Input: part model. Units: mm. Frame: model coordinates. Face numbers are marked on the shaded views. A direction names the side the tool comes from. Coordinates: 2 decimals unless noted, no trailing zeros. Write each loop counter-clockwise with the first axis right and the second up, starting at its lowest first coordinate (ties: lowest second). Pieces come first, ordered by that corner, then holes.
1) Pin query (flat end, axial travel): pin 1 Ø0.9 at (x, y) = (-39.5, 23) entering from +Z; pin 2 Ø2 at (y, z) = (-8.5, 6) entering from +X; pin 3 Ø0.6 at (y, z) = (42, 1) entering from +X. Return the tip coordinate at first contact, or that it passes through.
2) Section query C-C (z = 10.5). Output: boundary loops of the cut face in (x, y), then the cut area to 3 significant figures.
3) Section query D-D (y = 33.5). Output: boundary loops of the cut face in (x, z), then the cut area to 3 significant figures.
4) Set-up query: the marked faces 1 and 2. Return all of +Z, -Z, +X, -X, +Y, -Y with unobstructed straight access to the full face (end or side cutting, diameter ignored); none if empty.
5) Section query A-A (x = 0). Output: boundary loops of the cut face in (y, z), then the cut area to 3 significant figures.
6) Line query: L1, parallel to Z at x = 40, y = 0; L2, parallel to Y at x = -26, z = 1.75; L3, parallel to X at y = 5.5, z = 6.75. Output: solid intervals per line, ascending.
Autodesk Fusion 360 part; units mm, degrees
sketch "Sketch1" plane through (0, 0, 0) normal (0, 0, 1) x (1, 0, 0)
  circle A0 centre (0, 0) radius 38.1
  circle A1 centre (0, 0) radius 46 construction
  circle A2 centre (0, 46) radius 4
  line L0 (-3.9962, 45.8261) -> (-3.9962, 37.8898)
  line L1 (3.9962, 45.8261) -> (3.9962, 37.8898)
  circle A3 centre (0, 46) radius 1.5
  line L2 (-19.4522, 41.6847) -> (-15.4841, 34.8117)
  line L3 (-26.3739, 37.6884) -> (-22.4057, 30.8155)
  circle A4 centre (-23, 39.8372) radius 4
  circle A5 centre (-23, 39.8372) radius 1.5
  line L4 (-37.6884, 26.3739) -> (-30.8155, 22.4057)
  line L5 (-41.6847, 19.4522) -> (-34.8117, 15.4841)
  circle A6 centre (-39.8372, 23) radius 4
  circle A7 centre (-39.8372, 23) radius 1.5
  line L6 (-45.8261, 3.9962) -> (-37.8898, 3.9962)
  line L7 (-45.8261, -3.9962) -> (-37.8898, -3.9962)
  circle A8 centre (-46, 0) radius 4
  circle A9 centre (-46, 0) radius 1.5
  line L8 (-41.6847, -19.4522) -> (-34.8117, -15.4841)
  line L9 (-37.6884, -26.3739) -> (-30.8155, -22.4057)
  circle A10 centre (-39.8372, -23) radius 4
  circle A11 centre (-39.8372, -23) radius 1.5
  line L10 (-26.3739, -37.6884) -> (-22.4057, -30.8155)
  line L11 (-19.4522, -41.6847) -> (-15.4841, -34.8117)
  circle A12 centre (-23, -39.8372) radius 4
  circle A13 centre (-23, -39.8372) radius 1.5
  line L12 (-3.9962, -45.8261) -> (-3.9962, -37.8898)
  line L13 (3.9962, -45.8261) -> (3.9962, -37.8898)
  circle A14 centre (0, -46) radius 4
  circle A15 centre (0, -46) radius 1.5
  line L14 (19.4522, -41.6847) -> (15.4841, -34.8117)
  line L15 (26.3739, -37.6884) -> (22.4057, -30.8155)
  circle A16 centre (23, -39.8372) radius 4
  circle A17 centre (23, -39.8372) radius 1.5
  line L16 (37.6884, -26.3739) -> (30.8155, -22.4057)
  line L17 (41.6847, -19.4522) -> (34.8117, -15.4841)
  circle A18 centre (39.8372, -23) radius 4
  circle A19 centre (39.8372, -23) radius 1.5
  line L18 (45.8261, -3.9962) -> (37.8898, -3.9962)
  line L19 (45.8261, 3.9962) -> (37.8898, 3.9962)
  circle A20 centre (46, 0) radius 4
  circle A21 centre (46, 0) radius 1.5
  line L20 (41.6847, 19.4522) -> (34.8117, 15.4841)
  line L21 (37.6884, 26.3739) -> (30.8155, 22.4057)
  circle A22 centre (39.8372, 23) radius 4
  circle A23 centre (39.8372, 23) radius 1.5
  line L22 (26.3739, 37.6884) -> (22.4057, 30.8155)
  line L23 (19.4522, 41.6847) -> (15.4841, 34.8117)
  circle A24 centre (23, 39.8372) radius 4
  circle A25 centre (23, 39.8372) radius 1.5
  dimension "d374" = 76.2
  dimension "d375" = 92
  dimension "d376" = 8
  dimension "d377" = 3
  dimension "d379" = 360
extrude "Extrude1" add sketch "Sketch1" along normal blind 2 contours A0 | A0 L18 L19 A20 | A0 L20 L21 A22 | A20 | A0 L16 L17 A18 | A22 | A18 | A0 L22 L23 A24 | A0 L14 L15 A16 | A24 | A16 | A0 A2 L0 L1 | A0 L12 L13 A14 | A2 | A14 | A0 L2 L3 A4 | A0 L10 L11 A12 | A4 | A12 | A0 L4 L5 A6 | A0 L8 L9 A10 | A6 | A10 | A0 L6 L7 A8 | A8 | A3 | A5 | A7 | A9 | A11 | A13 | A15 | A17 | A19 | A21 | A23 | A25
extrude "Extrude2" add sketch "Sketch1" along normal blind 10 from surface at 2 contours A0
extrude "Extrude3" add sketch "Sketch1" along normal blind 3 from surface at 2 contours A3 | A5 | A7 | A9 | A11 | A13 | A15 | A17 | A19 | A21 | A23 | A25
equation "d374 = mmt_id"
equation "mmt_id = 76.2 mm"
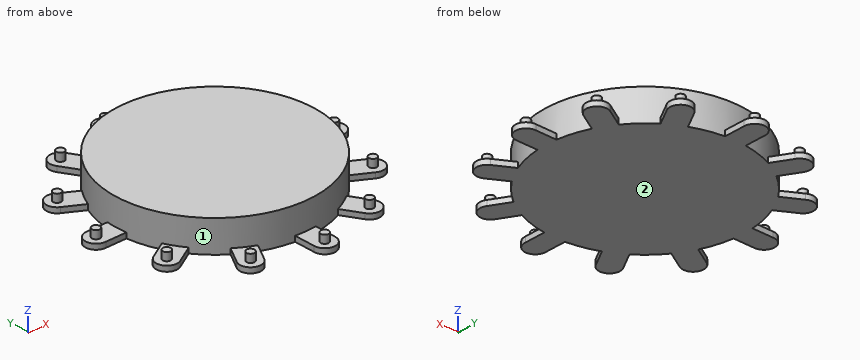
Answer:
1. pin 1: stops at z = 5
1. pin 2: stops at x = 37.35
1. pin 3: stops at x = 26.54
2. outline: circle Ø76.2 at (0, 0)
2. area: 4,560 mm2
3. outline: (-23.96, 0) - (23.96, 0) - (23.96, 2) - (18.15, 2) - (18.15, 12) - (-18.15, 12) - (-18.15, 2) - (-23.96, 2) - close
3. area: 459 mm2
4. face 1: +Z
4. face 2: -Z, +X, -X, +Y, -Y
5. outline: (-50, 0) - (50, 0) - (50, 2) - (47.5, 2) - (47.5, 5) - (44.5, 5) - (44.5, 2) - (38.1, 2) - (38.1, 12) - (-38.1, 12) - (-38.1, 2) - (-44.5, 2) - (-44.5, 5) - (-47.5, 5) - (-47.5, 2) - (-50, 2) - close
5. area: 980 mm2
6. L1: z = 0 to 2
6. L2: y = -42.48 to -37.04, -27.85 to 27.85, 37.04 to 42.48
6. L3: x = -37.7 to 37.7
